from build123d import *

# Parameters (mm, degrees)
SKETCH_1_R          = 9
EXTRUDE_1_DEPTH     = 48
EXTRUDE_2_DEPTH     = 3.5
SKETCH_3_R          = 11.75
EXTRUDE_3_DEPTH     = 3.5
SKETCH_4_R          = 8
CUT_EXTRUDE_1_DEPTH = 1.5
FILLET_1_R          = 0.75


with BuildPart() as part:
    # 草图1 → 凸台-拉伸1 (new body)
    with BuildSketch(Plane.XY):
        Circle(SKETCH_1_R)
    extrude(amount=EXTRUDE_1_DEPTH)

    # 草图2 → 凸台-拉伸2 (add)
    with BuildSketch(Plane(origin=(0, 0, 0), x_dir=(-1, 0, 0), z_dir=(0, 0, -1))):
        Polygon((-10.5, 4.349242405), (-10.5, -4.349242405), (-4.349242405, -10.5), (4.349242405, -10.5), (10.5, -4.349242405), (10.5, 4.349242405), (4.349242405, 10.5), (-4.349242405, 10.5), align=None)
    extrude(amount=-EXTRUDE_2_DEPTH)

    # 草图3 → 凸台-拉伸3 (add)
    with BuildSketch(Plane.XY.offset(3.5)):
        Circle(SKETCH_3_R)
    extrude(amount=EXTRUDE_3_DEPTH)

    # 草图4 → 切除-拉伸1 (cut)
    with BuildSketch(Plane.XY.offset(48)):
        Circle(SKETCH_4_R)
        with BuildLine():
            Line((6.633249581, -3.5), (0.25, -3.5))
            Line((0.25, -3.5), (0.25, 3.5))
            Line((0.25, 3.5), (6.633249581, 3.5))
            ThreePointArc((6.633249581, 3.5), (7.5, 0), (6.633249581, -3.5))
        make_face(mode=Mode.SUBTRACT)
        with BuildLine():
            Line((-0.25, -3.5), (-0.25, 3.5))
            Line((-0.25, 3.5), (-6.633249581, 3.5))
            ThreePointArc((-6.633249581, 3.5), (-7.5, 0), (-6.633249581, -3.5))
            Line((-6.633249581, -3.5), (-0.25, -3.5))
        make_face(mode=Mode.SUBTRACT)
    extrude(amount=-CUT_EXTRUDE_1_DEPTH, mode=Mode.SUBTRACT)

    # 圆角1
    fillet_1_edges = [part.edges().sort_by_distance(p)[0] for p in [
        (-3.44162479, 3.5, 46.5),
        (-3.44162479, -3.5, 48),
        (-7.5, 0, 48),
        (-0.25, 0, 48),
        (0.25, 0, 48),
        (3.44162479, -3.5, 48),
        (7.5, 0, 48),
        (3.44162479, 3.5, 48),
        (-3.44162479, -3.5, 46.5),
        (3.44162479, -3.5, 46.5),
        (3.44162479, 3.5, 46.5),
        (-3.44162479, 3.5, 48),
    ]]
    fillet(fillet_1_edges, radius=FILLET_1_R - 0.0001)  # a hair under: the kernel refuses the full size


solid = part.part
Source: CAD feature listing. Evaluate the final solid. Frame: model axes, mm. A direction names the side the tool comes from. Round coordinates to 2 decimals unless told otherwise and drop trailing zeros. Loops run counter-clockwise (first coordinate to the right, second up) from the corner with the lowest first, then second, coordinate; pieces in that order, holes last.
Q1. Section A-A, the plane y = 0. Return loops of the section in (x, z), plus the area to 3 significant figures.
Q2. Mould query, pull axis Y, two halves, no side actions, for faces 6 (the face through (-1.73, -7.81, 47.26)), 7 (the face through (0, -10.5, 2)), 8 (the face through (4, 0, 48)), 9 (the face through (-7.5, 0.1, 46.9)). Classes: pulls with the +Y half, pulls with the -Y half, needs draft (parallel to the pull), parting line crosses it, or undercut.
Q3. Section C-C, the plane z = 12. Return loops of the section in (x, y), plus the area to 3 significant figures.
Q4. Ray query, line 1 (Y direction, x = 0, z = 46.85); line 2 (Z direction, x = -5.5, y = 9); line 3 (X direction, y = -2.25, z = 3). Return the intervals inside material, ascending.
Q5. Access query for faces 1 (the face through (0, 10.5, 2)), 2 (the face through (0, -1, 46.5)), 3 (the face through (-10.5, 0, 2)), 4 (the face through (10.5, 0, 2)), 5 (the face through (7.38, 7.47, 1.73)). Directions: +Z, -Z, +X, -X, +Y, -Y. A direction counts if a zero-diameter tool reaches every point of the face in a straight line with its end or side. Return the directions, or none.
Q6. First-contact query: P1, Ø1, axis at x = 3, y = -1, coming from the -Z side; P2, Ø1.8, axis at x = 2, z = 1.5, coming from the -Y side; P3, Ø6, axis at x = 8, z = 10.5, coming from the +Y side; P4, Ø1.8, axis at y = 0, z = 1, coming from the +X side. Flat tips, straight axial feed; report the tip coordinate or a pass-through.
Solutions:
1. outline: (-11.75, 3.5) - (-10.5, 3.5) - (-10.5, 0) - (10.5, 0) - (10.5, 3.5) - (11.75, 3.5) - (11.75, 7) - (9, 7) - (9, 48) - (8, 48) - (8, 46.5) - (7.5, 46.5) - (7.5, 47.25) arc R0.75 ccw to (6.75, 48) - (1, 48) arc R0.75 ccw to (0.25, 47.25) - (0.25, 46.5) - (-0.25, 46.5) - (-0.25, 47.25) arc R0.75 ccw to (-1, 48) - (-6.75, 48) arc R0.75 ccw to (-7.5, 47.25) - (-7.5, 46.5) - (-8, 46.5) - (-8, 48) - (-9, 48) - (-9, 7) - (-11.75, 7) - close
1. area: 891 mm2
2. face 6: undercut
2. face 7: pulls with the -Y half
2. face 8: needs draft
2. face 9: undercut
3. outline: circle Ø18 at (0, 0)
3. area: 254 mm2
4. line 1: y = -9 to -8, 8 to 9
4. line 2: z = 0 to 7
4. line 3: x = -10.5 to 10.5
5. face 1: -Z, +X, -X, +Y
5. face 2: +Z
5. face 3: -Z, -X, +Y, -Y
5. face 4: -Z, +X, +Y, -Y
5. face 5: -Z, +X, +Y
6. P1: stops at z = 0
6. P2: stops at y = -10.5
6. P3: stops at y = 7.48
6. P4: stops at x = 10.5
